Build history of the part. All positions in model axes, mm. Round coordinates to 2 decimals unless told otherwise and drop trailing zeros. Loops run counter-clockwise (first coordinate to the right, second up) from the corner with the lowest first, then second, coordinate; pieces in that order, holes last. Notation, with made-up numbers: (-26, 61.5) - (-21, 61.5) arc R16 ccw to (-21, 87.5) - close; hole circle Ø11 at (-9, -37.5). An arc over 180 degrees is marked (long way). Put each result on its own line as item: value. Start each with the question number.
from build123d import *

# Parameters (mm, degrees)
SKIZZE1_R                       = 12.5
SKIZZE1_R_2                     = 2.5
AUFSATZ_LINEAR_AUSTRAGEN1_DEPTH = 2
SKIZZE2_W                       = 1
SKIZZE2_H                       = 6
SCHNITT_LINEAR_AUSTRAGEN1_DEPTH = 2
KREISMUSTER1_COUNT              = 31


with BuildPart() as part:
    # Skizze1 → Aufsatz-Linear austragen1 (new body)
    with BuildSketch(Plane.XY):
        Circle(SKIZZE1_R)
        Circle(SKIZZE1_R_2, mode=Mode.SUBTRACT)
    extrude(amount=AUFSATZ_LINEAR_AUSTRAGEN1_DEPTH)

    # Skizze2 → Schnitt-Linear austragen1 (cut)
    with BuildSketch(Plane.XY.offset(2)):
        with Locations((0, 9)):
            Rectangle(SKIZZE2_W, SKIZZE2_H)
    schnitt_linear_austragen1 = extrude(amount=-SCHNITT_LINEAR_AUSTRAGEN1_DEPTH, mode=Mode.SUBTRACT)

    # Kreismuster1: Schnitt-Linear austragen1 ×31 about axis
    kreismuster1_axis = Axis((0, 0, 0), (0, 0, 1))
    for i in range(1, KREISMUSTER1_COUNT):
        add(schnitt_linear_austragen1.rotate(kreismuster1_axis, i * 360 / KREISMUSTER1_COUNT), mode=Mode.SUBTRACT)


solid = part.part
Item 1: Slice it at A-A (y = 2). Give the cut face in (x, z).
Item 2: Slice it at B-B (z = 0.55). Give the number of separate pieces and of enclosed holes in the cut face, plus the area to 3 significant figures.
Item 3: Slice it at C-C (y = -9.75). Give the cut face in (x, z).
Item 4: Drill centre lines: probe 1 along Y at (x, z) = (0, 1.15); probe 2 along X at (y, z) = (10.5, 0.1); probe 3 along X at (y, z) = (-11, 0.2). Where is each one in solid material? Low to high. Write a range as [from, to].
Item 5: Drop flat-ended pins along their axis: pin 1 Ø1 at (y, z) = (2, 0.5) entering from -X; pin 2 Ø10 at (x, y) = (0.5, -7) entering from -Z; pin 3 Ø3 at (x, y) = (0, 0) entering from -Z. Give the stop position or say it passes through.
Computed values:
1. outline: (-12.34, 0) - (-11.83, 0) - (-11.83, 2) - (-12.34, 2) - close; (-9.75, 0) - (-6.84, 0) - (-6.84, 2) - (-9.75, 2) - close; (-5.66, 0) - (-1.5, 0) - (-1.5, 2) - (-5.66, 2) - close; (1.5, 0) - (5.66, 0) - (5.66, 2) - (1.5, 2) - close; (6.84, 0) - (9.75, 0) - (9.75, 2) - (6.84, 2) - close; (11.83, 0) - (12.34, 0) - (12.34, 2) - (11.83, 2) - close
2. separate pieces: 1
2. enclosed holes: 32
2. area: 285 mm^2
3. outline: (-7.82, 0) - (-5.98, 0) - (-5.98, 2) - (-7.82, 2) - close; (-4.84, 0) - (-3.58, 0) - (-3.58, 2) - (-4.84, 2) - close; (-2.54, 0) - (-1.49, 0) - (-1.49, 2) - (-2.54, 2) - close; (-0.49, 0) - (0.49, 0) - (0.49, 2) - (-0.49, 2) - close; (1.49, 0) - (2.54, 0) - (2.54, 2) - (1.49, 2) - close; (3.58, 0) - (4.84, 0) - (4.84, 2) - (3.58, 2) - close; (5.98, 0) - (7.82, 0) - (7.82, 2) - (5.98, 2) - close
4. probe 1: y = [-12.5, -2.5], [2.5, 6], [12, 12.5]
4. probe 2: x = [-6.78, -5.05], [-3.96, -2.67], [-1.65, -0.5], [0.5, 1.65], [2.67, 3.96], [5.05, 6.78]
4. probe 3: x = [-5.94, -3.98], [-2.93, -1.62], [-0.62, 0.62], [1.62, 2.93], [3.98, 5.94]
5. pin 1: stops at x = -12.41
5. pin 2: stops at z = 0
5. pin 3: passes through
